Can you work these out from the model? Positions are in its coordinate system, mm. Face numbers are marked on the shaded views. A direction names the side the tool comes from. Round coordinates to 2 decimals unless told otherwise and drop trailing zeros. Loops run counter-clockwise (first coordinate to the right, second up) from the corner with the lowest first, then second, coordinate; pieces in that order, holes last. Notation, with made-up numbers: (-29, -15.75) -> (-7, -15.75) arc R27 cw to (-7, 20.25) -> close; hole circle Ø9 at (-35.75, -15.5). An arc over 180 degrees is marked (long way). Use a Markdown table: item, result.
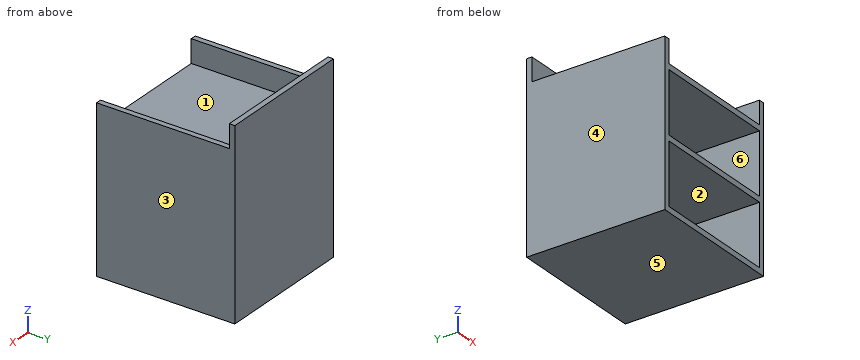
from build123d import *

# Parameters (mm, degrees)
F0_W      = 300
F0_H      = 300
F1_DEPTH  = 300
F2_T      = -12
F3_W      = 276
F3_H      = 12
F4_DEPTH  = 288
F5_W      = 300
F5_H      = 12
F6_DEPTH  = 100
F7_W      = 12
F7_H      = 288
F8_DEPTH  = 50
F9_W      = 12
F9_H      = 288
F10_DEPTH = 50


with BuildPart() as f1:
    # F0 (on Front) → F1 (new body)
    with BuildSketch(Plane.XZ):
        Rectangle(F0_W, F0_H)
    extrude(amount=-F1_DEPTH)

    # F2
    f2_openings = [f1.faces().sort_by_distance(p)[0] for p in [
        (0, 0, 0),
    ]]
    offset(amount=F2_T, openings=f2_openings)

    # F3 (on face) → F4 (join)
    with BuildSketch(Plane.XZ.offset(-288)):
        Rectangle(F3_W, F3_H)
    extrude(amount=F4_DEPTH)

    # F5 (on face) → F6 (join)
    with BuildSketch(Plane.XY.offset(150)):
        with Locations((0, 294)):
            Rectangle(F5_W, F5_H)
    extrude(amount=F6_DEPTH)

    # F7 (on face) → F8 (join)
    with BuildSketch(Plane.XY.offset(150)):
        with Locations((-144, 144)):
            Rectangle(F7_W, F7_H)
    extrude(amount=F8_DEPTH)

    # F9 (on face) → F10 (join)
    with BuildSketch(Plane.XY.offset(150)):
        with Locations((144, 144)):
            Rectangle(F9_W, F9_H)
    extrude(amount=F10_DEPTH)


solid = f1.part
1. I want a section at A-A (y = 130). Please give me the cut outline in (x, z), plus the area to 3 significant figures.
Answer sheet:
| item | result |
|---|---|
| outline | (-150, -150) -> (150, -150) -> (150, 200) -> (138, 200) -> (138, 150) -> (-138, 150) -> (-138, 200) -> (-150, 200) -> close; hole (-138, -138) -> (138, -138) -> (138, -6) -> (-138, -6) -> close; hole (-138, 6) -> (138, 6) -> (138, 138) -> (-138, 138) -> close |
| area | 18,300 mm² |
2. Will these pins go through, and if not, where does the flat tip stop? pin 1 Ø13 at (x, y) = (-142.5, 214) entering from +Z; pin 2 Ø8 at (x, z) = (-59, -73) entering from -Y.
Answer sheet:
| item | result |
|---|---|
| pin 1 | stops at z = 200 |
| pin 2 | stops at y = 288 |
3. Which directions (+Z, -Z, +X, -X, +Y, -Y) give clear straight access to the entire face, cutting with the end or side of a thin tool? Please do the marked faces 1, 2 and 3.
Answer sheet:
| item | result |
|---|---|
| face 1 | +Z, -Y |
| face 2 | -Y |
| face 3 | +Z, -Z, +X, +Y, -Y |
4. I need wall thicknesses on line 1 (Z direction, x = 87.5, y = 225); line 2 (X direction, y = 146, z = -71); line 3 (Y direction, x = 136.5, z = 230). Which ranges of each line are inside material? Lowest first, please.
Answer sheet:
| item | result |
|---|---|
| line 1 | z = -150 to -138, -6 to 6, 138 to 150 |
| line 2 | x = -150 to -138, 138 to 150 |
| line 3 | y = 288 to 300 |
5. I want a section at B-B (z = 39). Please give me the cut outline in (x, y), plus the area to 3 significant figures.
Answer sheet:
| item | result |
|---|---|
| outline | (-150, 0) -> (-138, 0) -> (-138, 288) -> (138, 288) -> (138, 0) -> (150, 0) -> (150, 300) -> (-150, 300) -> close |
| area | 10,500 mm² |
6. If we mould it in two halves opening along X, with no side actions, what happens to the marked faces 4, 5 and 6? For each: +X half, -X half, draft (parallel to the pull), parting line (faces both ways), or undercut.
Answer sheet:
| item | result |
|---|---|
| face 4 | -X half |
| face 5 | draft |
| face 6 | undercut |
7. I want a section at C-C (x = -90.5). Please give me the cut outline in (y, z), plus the area to 3 significant figures.
Answer sheet:
| item | result |
|---|---|
| outline | (0, -150) -> (300, -150) -> (300, 250) -> (288, 250) -> (288, 150) -> (0, 150) -> (0, 138) -> (288, 138) -> (288, 6) -> (0, 6) -> (0, -6) -> (288, -6) -> (288, -138) -> (0, -138) -> close |
| area | 15,200 mm² |
8. I want a section at D-D (z = 210). Please give me the cut outline in (x, y).
Answer sheet:
| item | result |
|---|---|
| outline | (-150, 288) -> (150, 288) -> (150, 300) -> (-150, 300) -> close |
